from build123d import *

# Parameters (mm, degrees)
EXTRUDE_1_DEPTH     = 6
SKETCH_2_W          = 6
SKETCH_2_H          = 8
SKETCH_2_R          = 1.65
EXTRUDE_2_DEPTH     = 2
EXTRUDE_START       = -32
SKETCH_3_W          = 6
SKETCH_3_H          = 12
EXTRUDE_3_DEPTH     = 4
CUT_EXTRUDE_1_REACH = 68.837
SKETCH_4_R          = 5.15


with BuildPart() as part:
    # 草图1 → 凸台-拉伸1 (new body)
    with BuildSketch(Plane.XY.offset(228)):
        with BuildLine():
            Line((25.153300859, 23.921391565), (19.791421356, 18.559512062))
            Line((19.791421356, 18.559512062), (12.208578644, 18.559512062))
            Line((12.208578644, 18.559512062), (12.208578644, 16.380432911))
            Line((12.208578644, 16.380432911), (14.08992832, 14.6918887))
            Line((14.08992832, 14.6918887), (18.591338638, 14.6918887))
            Line((18.591338638, 14.6918887), (24.706637775, 9.203300859))
            Line((24.706637775, 9.203300859), (28.187867966, 9.203300859))
            Line((28.187867966, 9.203300859), (35.812132034, 9.203300859))
            Line((35.812132034, 9.203300859), (41.203300859, 3.812132034))
            Line((41.203300859, 3.812132034), (41.203300859, -3.812132034))
            Line((41.203300859, -3.812132034), (35.812132034, -9.203300859))
            Line((35.812132034, -9.203300859), (28.187867966, -9.203300859))
            Line((28.187867966, -9.203300859), (24.706637775, -9.203300859))
            Line((24.706637775, -9.203300859), (18.591338638, -14.6918887))
            Line((18.591338638, -14.6918887), (14.08992832, -14.6918887))
            Line((14.08992832, -14.6918887), (12.208578644, -16.380432911))
            Line((12.208578644, -16.380432911), (12.187867966, -18.509512062))
            Line((12.187867966, -18.509512062), (19.812132034, -18.509512062))
            Line((19.812132034, -18.509512062), (25.203300859, -23.900680887))
            Line((25.203300859, -23.900680887), (25.203300859, -31.524944955))
            Line((25.203300859, -31.524944955), (19.812132034, -36.91611378))
            Line((19.812132034, -36.91611378), (12.187867966, -36.91611378))
            Line((12.187867966, -36.91611378), (0, -36.91611378))
            Line((0, -36.91611378), (0, -40.91611378))
            Line((0, -40.91611378), (22.203300859, -40.91611378))
            ThreePointArc((22.203300859, -40.91611378), (38.466756826, -34.179569747), (45.203300859, -17.91611378))
            Line((45.203300859, -17.91611378), (45.203300859, 17.86611378))
            ThreePointArc((45.203300859, 17.86611378), (38.466756826, 34.129569747), (22.203300859, 40.86611378))
            Line((22.203300859, 40.86611378), (0, 40.86611378))
            Line((0, 40.86611378), (0, 36.86611378))
            Line((0, 36.86611378), (12.208578644, 36.86611378))
            Line((12.208578644, 36.86611378), (19.791421356, 36.86611378))
            Line((19.791421356, 36.86611378), (25.153300859, 31.504234277))
            Line((25.153300859, 31.504234277), (25.153300859, 23.921391565))
        make_face()
    extrude(amount=-EXTRUDE_1_DEPTH)

    # 草图2 → 凸台-拉伸2 (add)
    # profile 1 of 2: a face of its own
    with BuildSketch(Plane.ZY):
        with Locations((225, 44.86611378)):
            Rectangle(SKETCH_2_W, SKETCH_2_H)
        with Locations(Location((225, 44.86611378, 0), (0, 0, 270))):
            Circle(SKETCH_2_R, mode=Mode.SUBTRACT)
    # profile 2 of 2: a face of its own
    with BuildSketch(Plane.ZY):
        with Locations((225, -44.86611378)):
            Rectangle(SKETCH_2_W, SKETCH_2_H)
        with Locations(Location((225, -44.86611378, 0), (0, 0, 90))):
            Circle(SKETCH_2_R, mode=Mode.SUBTRACT)
    extrude(amount=-EXTRUDE_2_DEPTH)

    # 草图3 → 凸台-拉伸3 (add)
    with BuildSketch(Plane.ZY.offset(EXTRUDE_START)):
        with Locations((225, 42.86611378)):
            Rectangle(SKETCH_3_W, SKETCH_3_H)
        with Locations((225, -42.86611378)):
            Rectangle(SKETCH_3_W, SKETCH_3_H)
    extrude(amount=EXTRUDE_3_DEPTH)

    # 草图4 → 切除-拉伸1 (cut, up to next)
    with BuildSketch(Plane(origin=(0, 0, 222), x_dir=(-1, 0, 0), z_dir=(0, 0, -1)), mode=Mode.PRIVATE) as cut_extrude_1_sk1:
        with Locations((-34.116390274, 18.292236363)):
            Circle(SKETCH_4_R)
    cut_extrude_1_tool1 = extrude(cut_extrude_1_sk1.sketch, amount=-CUT_EXTRUDE_1_REACH, mode=Mode.PRIVATE) & part.part
    # 草图4 → 切除-拉伸1 (cut, up to next)
    with BuildSketch(Plane(origin=(0, 0, 222), x_dir=(-1, 0, 0), z_dir=(0, 0, -1)), mode=Mode.PRIVATE) as cut_extrude_1_sk2:
        with Locations(Location((-34.116390274, -18.292236363, 0), (0, 0, 180))):
            Circle(SKETCH_4_R)
    cut_extrude_1_tool2 = extrude(cut_extrude_1_sk2.sketch, amount=-CUT_EXTRUDE_1_REACH, mode=Mode.PRIVATE) & part.part
    add(cut_extrude_1_tool1.solids().sort_by_distance((34.11639, 18.292236, 222))[0], mode=Mode.SUBTRACT)
    add(cut_extrude_1_tool2.solids().sort_by_distance((34.11639, -18.292236, 222))[0], mode=Mode.SUBTRACT)


solid = part.part
The model under review builds one solid part; all positions refer to its coordinate system, in mm. A direction names the side the tool comes from. Give positions to 0.01 mm unless a question says otherwise; leave off trailing zeros. Order: outer loops, then holes, each group sorted by start corner. A loop starts at its lowest first (then second) coordinate and runs counter-clockwise, first axis right, second up. Notation, with made-up numbers: M 79,-1.5 L 120,-1.5 A29 cw 120,35.5 Z; hole C -29,24 d10. An arc over 180 degrees is marked long. Answer in a Markdown table with one row per item. Add a question column.
1. For pin 1 Ø2 at (y, z) = (-34.5, 223.5) entering from +X; pin 2 Ø1 at (x, z) = (34, 223) entering from +Y; pin 3 Ø1 at (x, z) = (21, 224) entering from +Y, all flat-tipped, find the tip position at first contact; note any pin that passes through.
2. Add section C-C on y = -12. State the section outline as (x, z) points, plus the area to 3 significant figures.
3. Add section A-A on x = 8. State the section outline as (y, z) points.
4. Mouldability with a two-part tool opening along Y and no side actions: class faces 4 (the flat face through (12, 40.866, 225)), 5 (the flat face through (13.162, -15.524, 225.042)), 6 (the flat face through (2, -43, 225)), 7 (the flat face through (30, -48.866, 225)) as released by +Y, released by -Y, zero draft, split by the parting line, or undercut.
5. To check wall thickness, follow line 1 along Y through (x, z) = (0.6, 225); line 2 along Y through (x, z) = (15, 225.4); line 3 along Y through (x, z) = (28.5, 226.2). State the ranges of each line that lie inside material, in increasing order.
6. Add section B-B on z = 225. Count the separate pieces of the cut face and the enclosed holes in it, plus the area to 3 significant figures.
7. Machinability: for faces 1 (the flat face through (32, -44, 225)), 2 (the flat face through (12, -40.916, 225)), 3 (the flat face through (22.5, -21.2, 225)), which of the approach directions +Z, -Z, +X, -X, +Y, -Y give a long, thin tool a straight path to every point of the face, cutting with its end or side? Answer none if there is none.
8. Add section D-D on y = 7. State the section outline as (x, z) points.
The answers:
| question | item | result |
|---|---|---|
| 1 | pin 1 | x = 39.12 |
| 1 | pin 2 | y = 37.9 |
| 1 | pin 3 | y = 40.87 |
| 2 | outline | M 21.59,222 L 45.2,222 L 45.2,228 L 21.59,228 Z |
| 2 | area | 142 mm2 |
| 3 | outline | M -40.92,222 L -36.92,222 L -36.92,228 L -40.92,228 Z; M 36.87,222 L 40.87,222 L 40.87,228 L 36.87,228 Z |
| 4 | face 4 | released by +Y |
| 4 | face 5 | undercut |
| 4 | face 6 | zero draft |
| 4 | face 7 | released by -Y |
| 5 | line 1 | -48.87 to -46.52, -43.22 to -36.92, 36.87 to 43.22, 46.52 to 48.87 |
| 5 | line 2 | -40.92 to -36.92, -18.51 to -14.69, 14.69 to 18.56, 36.87 to 40.87 |
| 5 | line 3 | -48.87 to -9.2, 9.2 to 48.87 |
| 6 | separate pieces | 3 |
| 6 | enclosed holes | 2 |
| 6 | area | 1,470 mm2 |
| 7 | face 1 | +Z, -Z, +X, -Y |
| 7 | face 2 | +Z, -Z, -Y |
| 7 | face 3 | +Z, -Z, -X |
| 8 | outline | M 38.02,222 L 45.2,222 L 45.2,228 L 38.02,228 Z |
